The figure shows three views and two pictorial views of one solid part (mm, origin at its lowest corner). Answer the questions. A direction names the side the tool comes from. Coordinates: 2 decimals unless noted, no trailing zeros. Order: outer loops, then holes, each group sorted by start corner. A loop starts at its lowest first (then second) coordinate and runs counter-clockwise, first axis right, second up. Notation, with made-up numbers: (6, 67) -> (39, 67) arc R19 ccw to (39, 71) -> close; hole circle Ø6 at (-33, -37.5). An arc over 180 degrees is marked (long way). Write item = value, one per line. Start each with the question number.
Q1. Straight lines are drawn through the part: L1, parallel to Z at x = 19, y = 66; L2, parallel to Y at x = 24, z = 36.5; L3, parallel to X at y = 82, z = 20.5. For each, find the intervals that lie inside material, in ascending order. Write a range as from..to.
Q2. The part is cut by section A-A, the plane x = 20. Determine the outline of the cut face in (y, z).
Q3. The part is cut by section C-C, the plane y = 56.5. Determine the outline of the cut face in (x, z).
Q4. The part is cut by section D-D, the plane z = 4. Determine the outline of the cut face in (x, y).
Q5. Which of the six approach directions +Z, -Z, +X, -X, +Y, -Y give full straight-line access (tool end or side, diameter ignored) to the marked faces 1, 2 and 3?
Q6. The part is cut by section B-B, the plane z = 20. Determine the outline of the cut face in (x, y), plus the area to 3 significant figures.
Q7. Flat-ended cylindrical pins translate along their axes: pin 1 (4 mm diameter, centred on x = 31, z = 5, fed in from +Y); pin 2 (3 mm diameter, centred on y = 57.5, z = 23.5, fed in from +X); pin 3 (3 mm diameter, centred on y = 84.5, z = 8.5, fed in from +X). Find the tip coordinate at first contact, or state that the pin passes through.
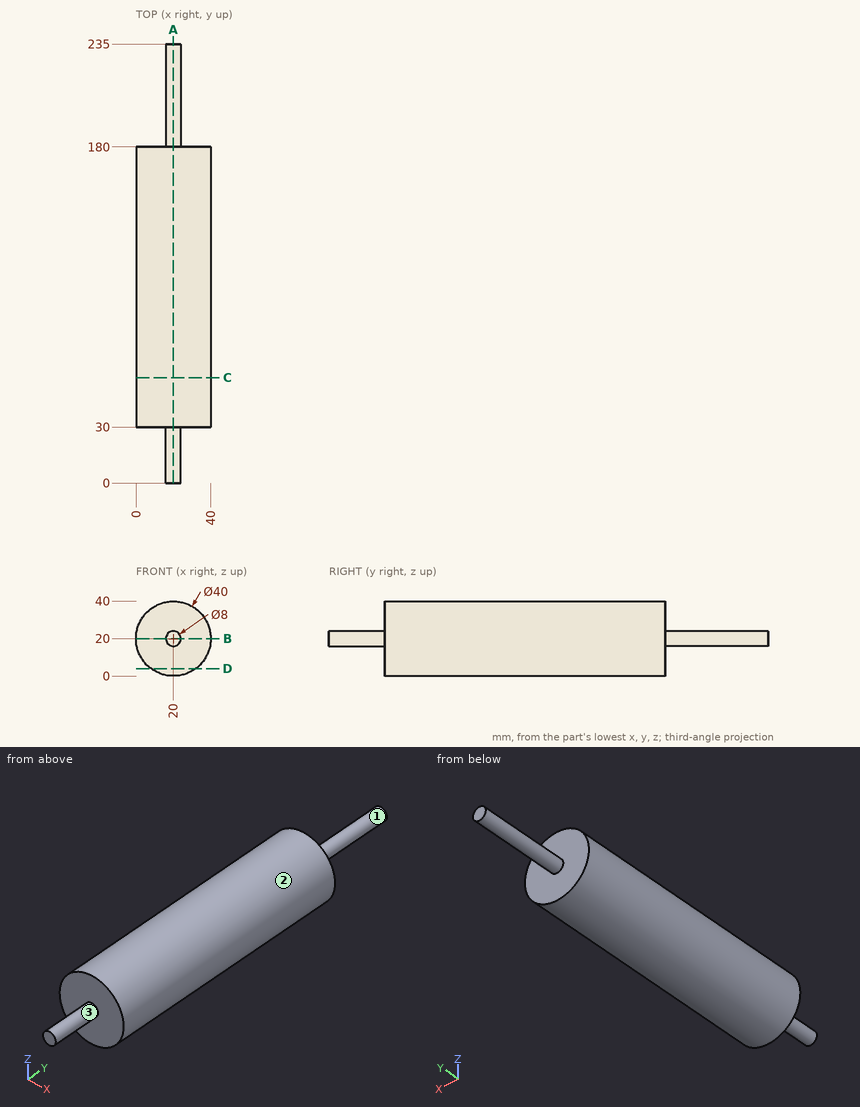
Model answer:
q1.L1 = 0.03..39.97
q1.L2 = 30..180
q1.L3 = 0.01..39.99
q2.outline = (0, 16) -> (30, 16) -> (30, 0) -> (180, 0) -> (180, 16) -> (235, 16) -> (235, 24) -> (180, 24) -> (180, 40) -> (30, 40) -> (30, 24) -> (0, 24) -> close
q3.outline = circle Ø40 at (20, 20)
q4.outline = (8, 30) -> (32, 30) -> (32, 180) -> (8, 180) -> close
q5.face_1 = +Y
q5.face_2 = +Y, -Y
q5.face_3 = -Y
q6.outline = (0, 30) -> (16, 30) -> (16, 0) -> (24, 0) -> (24, 30) -> (40, 30) -> (40, 180) -> (24, 180) -> (24, 235) -> (16, 235) -> (16, 180) -> (0, 180) -> close
q6.area = 6,680 mm2
q7.pin_1 = 180
q7.pin_2 = 39.9
q7.pin_3 = 37.32
